Input: dimensioned drawing with shaded views. Units: mm. Origin: part minimum x, y, z. Round coordinates to 2 decimals unless told otherwise and drop trailing zeros. Write each loop counter-clockwise with the first axis right and the second up, starting at its lowest first coordinate (ties: lowest second). Pieces come first, ordered by that corner, then holes. Notation, with made-up numbers: M 2,-6.5 L 39,-6.5 A22 ccw 39,6.5 Z; hole C 63,79 d7. An arc over 180 degrees is marked long. Use one line per item in the form item = value. Start each with the question number.
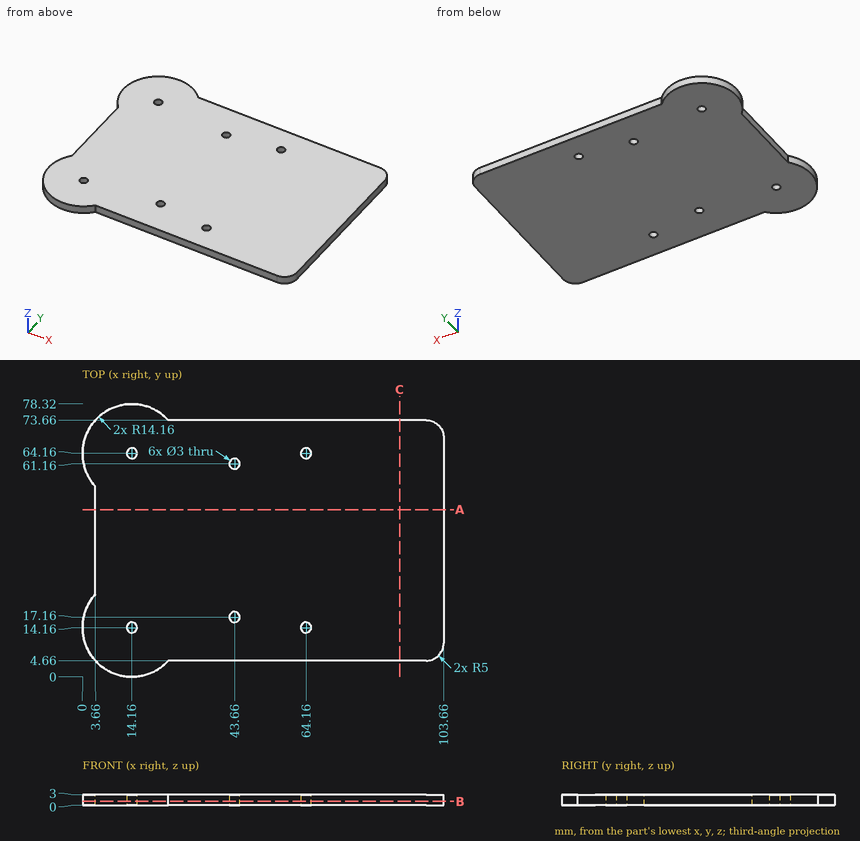
1. Ray query, probe 1 along X at (y, z) = (26, 1.65); probe 2 along X at (y, z) = (15, 0.65) (1 decimal); probe 3 along Y at (x, z) = (70, 2.5). Return the intervals inside material, ascending.
2. Section query B-B (z = 1.15). Return loops of the section in (x, y), then the cut area to 3 significant figures.
3. Contact query for flat-ended pins moving along their axis: pin 1 (2.5 mm diameter, centred on x = 14.16, y = 64.16, fed in from -Z); pin 2 (1.5 mm diameter, centred on x = 44, z = 2.5, fed in from -Y); pin 3 (1.5 mm diameter, centred on x = 47, z = 1, fed in from +Y); pin 4 (0.9 mm diameter, centred on y = 40, z = 2, fed in from -X). Output: stop coordinate, or through.
4. Section query A-A (y = 48). Return loops of the section in (x, z).
5. Section query C-C (x = 91). Return loops of the section in (y, z).
Checks:
q1.probe_1 = 3.66 to 103.66
q1.probe_2 = 0 to 12.9, 15.4 to 62.9, 65.4 to 103.7
q1.probe_3 = 4.66 to 73.66
q2.outline = M 3.66,23.66 A14.16 ccw 24.66,4.66 L 98.66,4.66 A5 ccw 103.66,9.66 L 103.66,68.66 A5 ccw 98.66,73.66 L 24.66,73.66 A14.16 ccw 3.66,54.66 Z; hole C 14.16,14.16 d3; hole C 14.16,64.16 d3; hole C 43.66,17.16 d3; hole C 43.66,61.16 d3; hole C 64.16,14.16 d3; hole C 64.16,64.16 d3
q2.area = 7,080 mm^2
q3.pin_1 = through
q3.pin_2 = 4.66
q3.pin_3 = 73.66
q3.pin_4 = 3.66
q4.outline = M 3.66,0 L 103.66,0 L 103.66,3 L 3.66,3 Z
q5.outline = M 4.66,0 L 73.66,0 L 73.66,3 L 4.66,3 Z
